from build123d import *

# Parameters (mm, degrees)
SKETCH1_R             = 7
SKETCH1_R_2           = 2
BOSS_EXTRUDE1_DEPTH   = 5
SKETCH1_R_3           = 38
SKETCH1_R_4           = 32.036519423
BOSS_EXTRUDE1_2_DEPTH = 5
BOSS_EXTRUDE2_DEPTH   = 1


with BuildPart() as part:
    # Sketch1 → Boss-Extrude1 (new, symmetric)
    with BuildSketch(Plane.XY):
        Circle(SKETCH1_R)
        Circle(SKETCH1_R_2, mode=Mode.SUBTRACT)
    extrude(amount=BOSS_EXTRUDE1_DEPTH, both=True)



with BuildPart() as body_2:
    # Sketch1 → Boss-Extrude1 2 (new, symmetric)
    with BuildSketch(Plane.XY):
        Circle(SKETCH1_R_3)
        Circle(SKETCH1_R_4, mode=Mode.SUBTRACT)
    extrude(amount=BOSS_EXTRUDE1_2_DEPTH, both=True)


with BuildPart() as part_1:
    add(part.part)

    add(body_2.part)  # Boss-Extrude2 merges body 2
    # Sketch1<4> → Boss-Extrude2 (add, symmetric)
    with BuildSketch(Plane.XY):
        with BuildLine():
            ThreePointArc((-6.659062866, -2.157980943), (-6.999999479, 0.002700877), (-6.657395614, 2.163118961))
            ThreePointArc((-6.657395614, 2.163118961), (-16.863954631, 11.260499688), (-30.468540556, 9.899828942))
            ThreePointArc((-30.468540556, 9.899828942), (-31.828331282, 3.646354962), (-31.918045732, -2.752622999))
            ThreePointArc((-31.918045732, -2.752622999), (-19.451242112, 4.455290106), (-6.659062866, -2.157980943))
        make_face()
        with BuildLine():
            ThreePointArc((-4.11012543, 5.666292346), (-2.160550113, 6.658229736), (0, 7))
            ThreePointArc((0, 7), (5.498123031, 19.518259711), (0, 32.036519423))
            ThreePointArc((0, 32.036519423), (-6.367605621, 31.39732752), (-12.481118599, 29.505258095))
            ThreePointArc((-12.481118599, 29.505258095), (-1.773531687, 19.875990918), (-4.11012543, 5.666292346))
        make_face()
        with BuildLine():
            ThreePointArc((4.118865652, 5.659942203), (5.664706075, 4.112311404), (6.657395614, 2.163118961))
            ThreePointArc((6.657395614, 2.163118961), (20.261981539, 0.802448215), (30.468540556, 9.899828942))
            ThreePointArc((30.468540556, 9.899828942), (27.892934581, 15.758260601), (24.20429022, 20.987875349))
            ThreePointArc((24.20429022, 20.987875349), (18.355139249, 7.828747841), (4.118865652, 5.659942203))
        make_face()
        with BuildLine():
            ThreePointArc((27.440192629, -16.534037778), (13.117631611, -15.037558663), (6.655724398, -2.16825569))
            ThreePointArc((6.655724398, -2.16825569), (5.661531003, -4.116681515), (4.114496766, -5.663118961))
            ThreePointArc((4.114496766, -5.663118961), (7.024470239, -19.02231944), (18.830593651, -25.918088654))
            ThreePointArc((18.830593651, -25.918088654), (23.606387238, -21.658186865), (27.440192629, -16.534037778))
        make_face()
        with BuildLine():
            ThreePointArc((-7.245318518, -31.206472667), (-10.247997062, -17.122470203), (-0.005401754, -6.999997916))
            ThreePointArc((-0.005401754, -6.999997916), (-2.165687487, -6.656560502), (-4.114496766, -5.663118961))
            ThreePointArc((-4.114496766, -5.663118961), (-15.920620178, -12.558888174), (-18.830593651, -25.918088654))
            ThreePointArc((-18.830593651, -25.918088654), (-13.303384916, -29.143756218), (-7.245318518, -31.206472667))
        make_face()
    extrude(amount=BOSS_EXTRUDE2_DEPTH, both=True)


solid = part_1.part
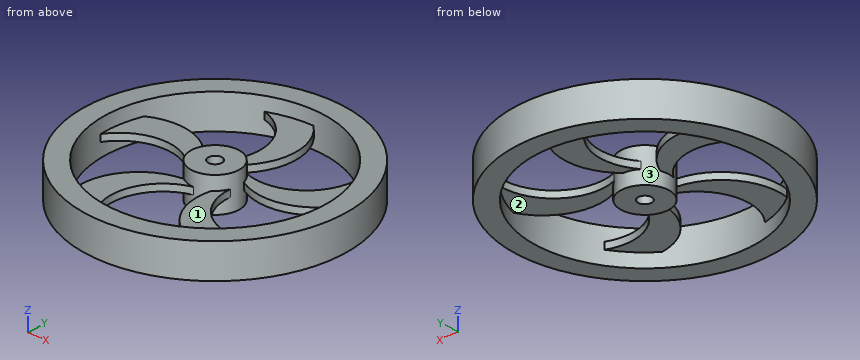
Geometry check sheet. Reference: the model listing, model coordinates, mm. Face numbers are marked on the shaded views. A direction names the side the tool comes from. Round coordinates to 2 decimals unless told otherwise and drop trailing zeros. Order: outer loops, then holes, each group sorted by start corner. A loop starts at its lowest first (then second) coordinate and runs counter-clockwise, first axis right, second up. Notation, with made-up numbers: (68, 7.25) - (101, 7.25) arc R18 cw to (101, 15.25) - close; hole circle Ø11 at (6, 6). An arc over 180 degrees is marked (long way). One line per question, with ' | ' between items. Start each with the question number.
(1) Sectioned sample at D-D on x = -3. Record the cut outline in (y, z).
(2) Sectioned sample at B-B on x = 13.5. Record the cut outline in (y, z), and give its area (3 significant figures).
(3) Access from +Z, -Z, +X, -X, +Y, -Y to the whole of each face (thin tool, end or side, straight path). Record for the marked faces 1, 2 and 3.
(4) Sectioned sample at A-A on z = -4. Record the cut outline in (x, y).
(5) Sectioned sample at C-C on y = -9. Record the cut outline in (x, z).
(6) Depth check by flat-ended pin: pin 1 Ø7 at (x, y) = (12.5, -19.5) entering from +Z; pin 2 Ø1 at (x, z) = (-18, -3) entering from +Y; pin 3 Ø6 at (x, z) = (-4, -1) entering from -Y. Enter the tip coordinate at first touch or a pass-through.
(7) Thickness scan on L1, parallel to Y at x = 0, z = 2.5; L2, parallel to Y at x = 0.5, z = 3; L3, parallel to X at y = 20.5, z = 0. Record the ranges inside material, lowest first. Write a range as [from, to].
Conclusion:
1) outline: (-37.88, -5) - (-31.9, -5) - (-31.9, 5) - (-37.88, 5) - close; (-8.22, -1) - (-6.32, -1) - (-6.32, -5) - (6.32, -5) - (6.32, -1) - (7.3, -1) - (7.3, 1) - (6.32, 1) - (6.32, 5) - (-6.32, 5) - (-6.32, 1) - (-8.22, 1) - close; (22.52, -1) - (31.9, -1) - (31.9, -5) - (37.88, -5) - (37.88, 5) - (31.9, 5) - (31.9, 1) - (22.52, 1) - close
2) outline: (-35.52, -5) - (-29.05, -5) - (-29.05, 5) - (-35.52, 5) - close; (-24.39, -1) - (-15.29, -1) - (-15.29, 1) - (-24.39, 1) - close; (0.04, -1) - (5.37, -1) - (5.37, 1) - (0.04, 1) - close; (29.05, -5) - (35.52, -5) - (35.52, 5) - (29.05, 5) - close | area: 158 mm2
3) face 1: +Z | face 2: -Z | face 3: none
4) outline: circle Ø76 at (0, 0); circle Ø14 at (0, 0); hole circle Ø64.07 at (0, 0); hole circle Ø4 at (0, 0)
5) outline: (-36.92, -5) - (-30.75, -5) - (-30.75, 5) - (-36.92, 5) - close; (-12.43, -1) - (-4.29, -1) - (-4.29, 1) - (-12.43, 1) - close; (3.78, -1) - (8.03, -1) - (8.03, 1) - (3.78, 1) - close; (30.75, -5) - (36.92, -5) - (36.92, 5) - (30.75, 5) - close
6) pin 1: stops at z = 1 | pin 2: stops at y = 33.73 | pin 3: stops at y = -37.99
7) L1: y = [-38, -32.04], [-7, -2], [2, 7], [32.04, 38] | L2: y = [-38, -32.03], [-6.98, -1.94], [1.94, 6.98], [32.03, 38] | L3: x = [-32, -24.62], [-2.01, 5.47], [24.24, 32]
